Source: CAD feature listing. Evaluate the final solid. Frame: model axes, mm. Face numbers are marked on the shaded views. A direction names the side the tool comes from. Round coordinates to 2 decimals unless told otherwise and drop trailing zeros.
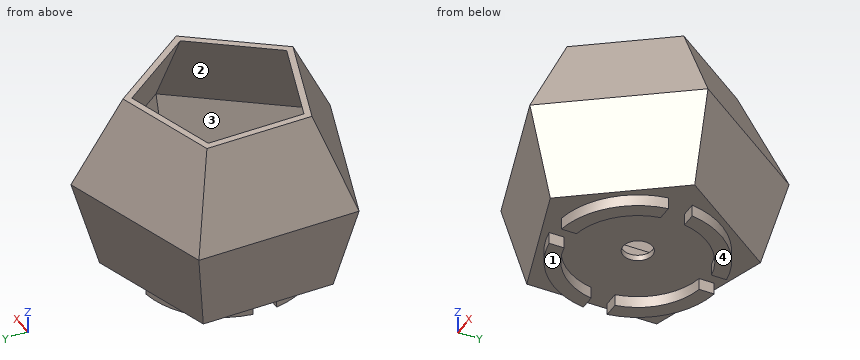
from build123d import *

# Parameters (mm, degrees)
VACIADO1_T              = -1
CROQUIS6_R              = 2.480361355
CORTAR_EXTRUIR1_DEPTH   = 10
SALIENTE_EXTRUIR1_DEPTH = 2


with BuildPart() as part:
    # Croquis2 → Recubrir1 section 0
    with BuildSketch(Plane.XY):
        with BuildLine():
            Line((18.541019662, 0), (5.729490169, 17.633557569))
            Line((5.729490169, 17.633557569), (-15, 10.89813792))
            Line((-15, 10.89813792), (-15, -10.89813792))
            Line((-15, -10.89813792), (5.729490169, -17.633557569))
            Line((5.729490169, -17.633557569), (18.541019662, 0))
        make_face()
    # Croquis3 → Recubrir1 section 1
    with BuildSketch(Plane.XY.offset(15)):
        with BuildLine():
            Line((22.867257584, 0), (7.066371208, 21.748054335))
            Line((7.066371208, 21.748054335), (-18.5, 13.441036768))
            Line((-18.5, 13.441036768), (-18.5, -13.441036768))
            Line((-18.5, -13.441036768), (7.066371208, -21.748054335))
            Line((7.066371208, -21.748054335), (22.867257584, 0))
        make_face()
    loft()

    # Croquis4 → section 1 of recubrir2
    with BuildSketch(Plane.XY.offset(30), mode=Mode.PRIVATE) as recubrir2_s1:
        with BuildLine():
            Line((15, 0), (4.635254916, 14.265847744))
            Line((4.635254916, 14.265847744), (-12.135254916, 8.816778784))
            Line((-12.135254916, 8.816778784), (-12.135254916, -8.816778784))
            Line((-12.135254916, -8.816778784), (4.635254916, -14.265847744))
            Line((4.635254916, -14.265847744), (15, 0))
        make_face()
    # loft from a face of the part (recubrir2)
    loft([part.faces().sort_by_distance((0, 0, 15))[0], recubrir2_s1.sketch])

    # Vaciado1
    vaciado1_openings = [part.faces().sort_by_distance(p)[0] for p in [
        (0, 0, 30),
    ]]
    offset(amount=VACIADO1_T, openings=vaciado1_openings, kind=Kind.INTERSECTION)

    # Croquis6 → Cortar-Extruir1 (cut)
    with BuildSketch(Plane(origin=(0, 0, 0), x_dir=(-1, 0, 0), z_dir=(0, 0, -1))):
        Circle(CROQUIS6_R)
    extrude(amount=-CORTAR_EXTRUIR1_DEPTH, mode=Mode.SUBTRACT)

    # Croquis7 → Saliente-Extruir1 (add)
    with BuildSketch(Plane(origin=(0, 0, 0), x_dir=(-1, 0, 0), z_dir=(0, 0, -1))):
        with BuildLine():
            Line((-2, 13.856406461), (-2, 11.324751653))
            ThreePointArc((-2, 11.324751653), (-8.131727984, 8.131727984), (-11.324751653, 2))
            Line((-11.324751653, 2), (-13.856406461, 2))
            ThreePointArc((-13.856406461, 2), (-9.899494937, 9.899494937), (-2, 13.856406461))
        make_face()
        with BuildLine():
            Line((2, 13.856406461), (2, 11.324751653))
            ThreePointArc((2, 11.324751653), (8.131727984, 8.131727984), (11.324751653, 2))
            Line((11.324751653, 2), (13.856406461, 2))
            ThreePointArc((13.856406461, 2), (9.899494937, 9.899494937), (2, 13.856406461))
        make_face()
        with BuildLine():
            Line((-13.856406461, -2), (-11.324751653, -2))
            ThreePointArc((-11.324751653, -2), (-8.131727984, -8.131727984), (-2, -11.324751653))
            Line((-2, -11.324751653), (-2, -13.856406461))
            ThreePointArc((-2, -13.856406461), (-9.899494937, -9.899494937), (-13.856406461, -2))
        make_face()
        with BuildLine():
            Line((11.324751653, -2), (13.856406461, -2))
            ThreePointArc((13.856406461, -2), (9.899494937, -9.899494937), (2, -13.856406461))
            Line((2, -13.856406461), (2, -11.324751653))
            ThreePointArc((2, -11.324751653), (8.131727984, -8.131727984), (11.324751653, -2))
        make_face()
    extrude(amount=SALIENTE_EXTRUIR1_DEPTH)


solid = part.part
1) Material intervals for line 1 (X direction, y = -2, z = 9); line 2 (Z direction, x = -8, y = 4); line 3 (Y direction, x = 0, z = 0.75), sorted ascending.
Taken from the geometry:
line 1: x = -17.1 to -16.07, 18.41 to 19.68
line 2: z = 0 to 1
line 3: y = -15.96 to -2.48, 2.48 to 15.96
2) Pull-direction query (X, two-part tool) for the marked faces 1 and 2; classes: released by +X, released by -X, zero draft, split by the parting line, or undercut.
Taken from the geometry:
face 1: zero draft
face 2: undercut
3) Reachability of the marked faces 3 and 4 from +Z, -Z, +X, -X, +Y, -Y: full face, straight path, thin tool, end or side. Return the list, or none.
Taken from the geometry:
face 3: none
face 4: -Z, +X, -X, +Y, -Y
4) Contact query for flat-ended pins moving along their axis: P1, Ø4, axis at x = 0, y = 0, coming from the -Z side; P2, Ø4, axis at x = 5.5, z = 9.5, coming from the -Y side; P3, Ø2, axis at y = 3, z = 6, coming from the -X side; P4, Ø0.6, axis at x = 13, z = -1, coming from the +Y side. Output: stop coordinate, or through.
Taken from the geometry:
P1: passes through
P2: stops at y = -20.67
P3: stops at x = -16.63
P4: stops at y = 5.89
